The listing builds one solid part. Answer for the finished solid, in the listing's coordinates (mm). Face numbers are marked on the shaded views. A direction names the side the tool comes from. Round coordinates to 2 decimals unless told otherwise and drop trailing zeros. Loops run counter-clockwise (first coordinate to the right, second up) from the corner with the lowest first, then second, coordinate; pieces in that order, holes last. Notation, with made-up numbers: (75.25, -8.75) - (101.25, -8.75) arc R30 cw to (101.25, 18.25) - close; hole circle Ø7 at (36.25, 3). An arc over 180 degrees is marked (long way). Write item = value, one per line. Start each with the question number.
1) Section A-A, the plane z = -18.25 is taken. Determine the outline of the cut face in (x, y) (3 decimals), and give its area (3 significant figures).
2) For a pull along Z with two mould halves and no side action, classify the marked faces 1, 2 and 3 as released by +Z, released by -Z, zero draft, split by the parting line, or undercut.
3) Section D-D, the plane x = 38.1 is taken. Determine the outline of the cut face in (y, z) (1 decimal), and give its area (3 significant figures).
4) Straight lines are drawn through the part: line 1 along Y through (x, z) = (38.1, -1.45); line 2 along Y through (x, z) = (40, -15.75) (3 decimals); line 3 along Z through (x, y) = (67.5, 36.5) (3 decimals). For each, find the intervals that lie inside material, in ascending order.
5) Section C-C, the plane y = 44.5 is taken. Determine the outline of the cut face in (x, z) (3 decimals).
6) Given pin 1 Ø8 at (x, y) = (28.5, 35.5) entering from +Z; pin 2 Ø10 at (y, z) = (34.5, -8.5) entering from -X, each flat-ended and moving along its own axis, determine where each tip first touches the part or whether it passes through.
7) Section B-B, the plane x = 15.5 is taken. Determine the outline of the cut face in (y, z) (3 decimals), and give its area (3 significant figures).
8) A tool of negligible diameter and unlimited length cuts with its end or side. For the marked faces 4 and 5, from which of +Z, -Z, +X, -X, +Y, -Y can it reach the whole face along a straight path? Write none if from no direction.
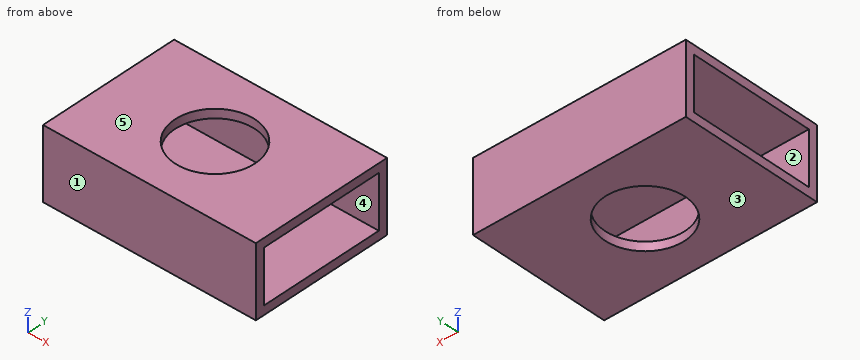
Autodesk Inventor part; units mm, degrees
ref_plane "YZ Plane" through (0, 0, 0) normal (1, 0, 0) x (0, 1, 0)
ref_plane "XZ Plane" through (0, 0, 0) normal (0, 1, 0) x (-1, 0, 0)
ref_plane "XY Plane" through (0, 0, 0) normal (0, 0, 1) x (1, 0, 0)
sketch "Sketch1" plane through (0, 0, 0) normal (1, 0, 0) x (0, 1, 0)
  line L0 (0, 0) -> (50.8, 0)
  line L1 (50.8, 0) -> (50.8, -25.4)
  line L2 (50.8, -25.4) -> (0, -25.4)
  line L3 (0, -25.4) -> (0, 0)
  line L4 (47.625, -22.225) -> (47.625, -3.175)
  line L5 (47.625, -3.175) -> (3.175, -3.175)
  line L6 (3.175, -3.175) -> (3.175, -22.225)
  line L7 (3.175, -22.225) -> (47.625, -22.225)
  dimension "d0" = 50.8
  dimension "d1" = 25.4
  dimension "d2" = 3.175
extrude "Extrusion1" add sketch "Sketch1" along normal blind 76.2
sketch "Sketch2" plane through (0, 0, 0) normal (0, 0, 1) x (1, 0, 0)
  circle A0 centre (38.1, 25.4) radius 14.2875
  point P0 (0, 0)
  dimension "d5" = 28.575
extrude "Extrusion2" cut sketch "Sketch2" against normal blind 76.2
properties part number "liftaxelbar"
Geometry check:
q1.outline = (0, 0) - (76.2, 0) - (76.2, 3.175) - (0, 3.175) - close; (0, 47.625) - (76.2, 47.625) - (76.2, 50.8) - (0, 50.8) - close
q1.area = 484 mm2
q2.face_1 = zero draft
q2.face_2 = undercut
q2.face_3 = released by -Z
q3.outline = (0, -25.4) - (11.1, -25.4) - (11.1, -22.2) - (3.2, -22.2) - (3.2, -3.2) - (11.1, -3.2) - (11.1, 0) - (0, 0) - close; (39.7, -25.4) - (50.8, -25.4) - (50.8, 0) - (39.7, 0) - (39.7, -3.2) - (47.6, -3.2) - (47.6, -22.2) - (39.7, -22.2) - close
q3.area = 262 mm2
q4.line_1 = 0 to 11.11, 39.69 to 50.8
q4.line_2 = 0 to 3.175, 47.625 to 50.8
q4.line_3 = -25.4 to -22.225, -3.175 to 0
q5.outline = (0, -25.4) - (76.2, -25.4) - (76.2, -22.225) - (0, -22.225) - close; (0, -3.175) - (76.2, -3.175) - (76.2, 0) - (0, 0) - close
q6.pin_1 = 0
q6.pin_2 = through
q7.outline = (0, -25.4) - (50.8, -25.4) - (50.8, 0) - (0, 0) - close; hole (3.175, -22.225) - (47.625, -22.225) - (47.625, -3.175) - (3.175, -3.175) - close
q7.area = 444 mm2
q8.face_4 = +X, -X
q8.face_5 = +Z, +X, -X, +Y, -Y
